For this review, take the finished solid that the model builds, in its own axes (mm). Give positions to 0.01 mm unless a question says otherwise; leave off trailing zeros. Order: outer loops, then holes, each group sorted by start corner. A loop starts at its lowest first (then second) coordinate and runs counter-clockwise, first axis right, second up.
from build123d import *

# Parameters (mm, degrees)
SKETCH1_W            = 190.87
SKETCH1_H            = 35
BOSS_EXTRUDE1_DEPTH  = 1.5
SKETCH2_R            = 21
CUT_EXTRUDE1_DEPTH   = 98.072597704
SKETCH3_W            = 25
SKETCH3_H            = 3
BOSS_EXTRUDE2_DEPTH  = 85
CHAMFER1_SIZE        = 5
CUT_EXTRUDE2_REACH   = 142.082
SKETCH4_R            = 5
CHAMFER2_SIZE        = 10
M4_CLEARANCE_HOLE1_D = 4.5
CHAMFER3_SIZE        = 2.5


with BuildPart() as part:
    # Sketch1 → Boss-Extrude1 (new, symmetric)
    with BuildSketch(Plane.XY):
        Rectangle(SKETCH1_W, SKETCH1_H)
    extrude(amount=BOSS_EXTRUDE1_DEPTH, both=True)

    # Sketch2 → Cut-Extrude1 (cut, through all)
    with BuildSketch(Plane.XY.offset(1.5)):
        with Locations((-2.565, 17.5)):
            Circle(SKETCH2_R)
    extrude(amount=-CUT_EXTRUDE1_DEPTH, mode=Mode.SUBTRACT)

    # Sketch3 → Boss-Extrude2 (add)
    with BuildSketch(Plane(origin=(0, 17.5, 0), x_dir=(1, 0, 0), z_dir=(0, 1, 0))):
        with Locations((-66.315, 0)):
            Rectangle(SKETCH3_W, SKETCH3_H)
    extrude(amount=BOSS_EXTRUDE2_DEPTH)

    # Chamfer1
    chamfer1_edges = [part.edges().sort_by_distance(p)[0] for p in [
        (-53.815, 102.5, 0),
        (-78.815, 102.5, 0),
    ]]
    chamfer(chamfer1_edges, length=CHAMFER1_SIZE)

    # Sketch4 → Cut-Extrude2 (cut, up to next)
    with BuildSketch(Plane.XY.offset(1.5), mode=Mode.PRIVATE) as cut_extrude2_sk1:
        with Locations((-66.315, 85)):
            Circle(SKETCH4_R)
    cut_extrude2_tool1 = extrude(cut_extrude2_sk1.sketch, amount=-CUT_EXTRUDE2_REACH, mode=Mode.PRIVATE) & part.part
    add(cut_extrude2_tool1.solids().sort_by_distance((-66.315, 85, 1.5))[0], mode=Mode.SUBTRACT)

    # Chamfer2
    chamfer2_edges = [part.edges().sort_by_distance(p)[0] for p in [
        (-53.815, 17.5, 0),
        (-78.815, 17.5, 0),
    ]]
    chamfer(chamfer2_edges, length=CHAMFER2_SIZE)

    # M4 Clearance Hole1 (through all)
    with Locations(Plane(origin=(0, 0, -1.5), x_dir=(-1, 0, 0), z_dir=(0, 0, -1))):
        with Locations((-89.185, 7.5), (-89.185, -7.5), (89.19, 7.5), (89.19, -7.5)):
            Hole(M4_CLEARANCE_HOLE1_D / 2)

    # Chamfer3
    # the kernel refuses this chamfer: 2.5 mm, written as the material it takes off along each edge
    with BuildSketch(Plane(origin=(18.435, 17.5, 8.379480144), x_dir=(-0.06371254293281461, -0.9979682920178548, 0), z_dir=(0, 0, -1))) as chamfer3_piece_1:
        with BuildLine():
            Line((2.675926803, 0), (-CHAMFER3_SIZE * 0.0637125429328, -CHAMFER3_SIZE * 0.997968292018))
            Line((-CHAMFER3_SIZE * 0.0637125429328, -CHAMFER3_SIZE * 0.997968292018), (0, 0))
            ThreePointArc((0, 0), (1.375635219, -0.042632078), (2.675926803, 0))
        make_face()
    extrude(amount=16.758960289, mode=Mode.SUBTRACT)
    with BuildSketch(Plane(origin=(-23.565, 17.5, -8.379480144), x_dir=(-1, 0, 0), z_dir=(0, 0, 1))) as chamfer3_piece_2:
        with BuildLine():
            Line((CHAMFER3_SIZE, 0), (-0.170490101, 2.670490101))
            ThreePointArc((-0.170490101, 2.670490101), (-0.045099756, 1.375556528), (0, 0))
            Line((0, 0), (CHAMFER3_SIZE, 0))
        make_face()
    extrude(amount=16.758960289, mode=Mode.SUBTRACT)


solid = part.part
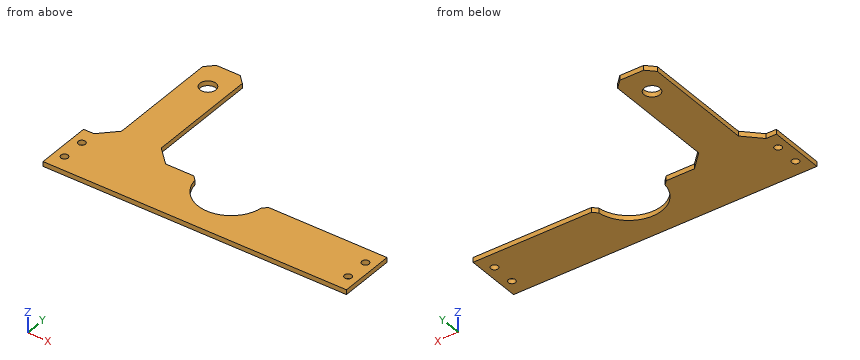
1) We need section A-A on y = 85. Give the boundary of the cut face in (x, z) (3 decimals), then the cut area to 3 significant figures.
Answer sheet:
outline: (-78.815, -1.5) - (-71.315, -1.5) - (-71.315, 1.5) - (-78.815, 1.5) - close; (-61.315, -1.5) - (-53.815, -1.5) - (-53.815, 1.5) - (-61.315, 1.5) - close
area: 45.0 mm2
2) We need section D-D on y = 7.5. Give the boundary of the cut face in (x, z) (3 decimals), then the cut area to 3 significant figures.
Answer sheet:
outline: (-95.435, -1.5) - (-91.44, -1.5) - (-91.44, 1.5) - (-95.435, 1.5) - close; (-86.94, -1.5) - (-21.031, -1.5) - (-21.031, 1.5) - (-86.94, 1.5) - close; (15.901, -1.5) - (86.935, -1.5) - (86.935, 1.5) - (15.901, 1.5) - close; (91.435, -1.5) - (95.435, -1.5) - (95.435, 1.5) - (91.435, 1.5) - close
area: 435 mm2
3) We need section B-B on y = -7.5. Give the boundary of the cut face in (x, z) (3 decimals).
Answer sheet:
outline: (-95.435, -1.5) - (-91.44, -1.5) - (-91.44, 1.5) - (-95.435, 1.5) - close; (-86.94, -1.5) - (86.935, -1.5) - (86.935, 1.5) - (-86.94, 1.5) - close; (91.435, -1.5) - (95.435, -1.5) - (95.435, 1.5) - (91.435, 1.5) - close
4) To check wall thickness, follow line 1 (Y direction, x = -89.19, z = 0); line 2 (X direction, y = 47, z = 0.5) (3 decimals); line 3 (Y direction, x = -62.5, z = -1.1). State the ranges of each line that lie inside material, in increasing order.
Answer sheet:
line 1: y = -17.5 to -9.75, -5.25 to 5.25, 9.75 to 17.5
line 2: x = -78.815 to -53.815
line 3: y = -17.5 to 81.77, 88.23 to 102.5
5) We need section C-C on z = -0.75. Count the separate pieces of the cut face and the enclosed holes in it, then the cut area to 3 significant figures.
Answer sheet:
separate pieces: 1
enclosed holes: 5
area: 8,040 mm2
6) Clearance check with flat-ended pins moving along their axes: pin 1 (2.5 mm diameter, centred on x = 89.185, y = 7.5, fed in from -Z); pin 2 (1.5 mm diameter, centred on x = -93, z = 0, fed in from +Y). State where each tip first meets the part, or that it passes through.
Answer sheet:
pin 1: passes through
pin 2: stops at y = 17.5
